Autodesk Inventor part; units mm, degrees
ref_plane "YZ Plane" through (0, 0, 0) normal (1, 0, 0) x (0, 1, 0)
ref_plane "XZ Plane" through (0, 0, 0) normal (0, 1, 0) x (-1, 0, 0)
ref_plane "XY Plane" through (0, 0, 0) normal (0, 0, 1) x (1, 0, 0)
sketch "スケッチ1" plane through (0, 0, 0) normal (0, 0, 1) x (1, 0, 0)
  circle A0 centre (0, 0) radius 1.5
  dimension "d0" = 3
extrude "押し出し1" add sketch "スケッチ1" along normal blind 18
sketch "スケッチ2" plane through (0, 0, 0) normal (0, 0, -1) x (-1, 0, 0)
  circle A0 centre (0, 0) radius 2.75
  dimension "d3" = 5.5
extrude "押し出し2" add sketch "スケッチ2" along normal blind 2
fillet "フィレット1" radius 2 1 edges at (2.75, 0, -2)
thread "ねじ1"
properties part number "ネジ鍋m3,18" material "鋼、高強度、低合金"
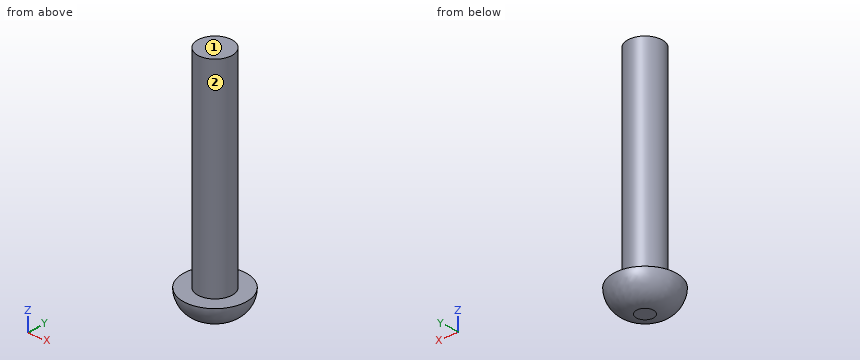
Read the model definition and answer for the solid it produces. Units are mm, in the model's axes. Face numbers are marked on the shaded views. A direction names the side the tool comes from. Coordinates: 2 decimals unless noted, no trailing zeros. Order: outer loops, then holes, each group sorted by start corner. A loop starts at its lowest first (then second) coordinate and runs counter-clockwise, first axis right, second up. Notation, with made-up numbers: (28, 3.25) -> (52, 3.25) arc R33 cw to (52, 38.25) -> close; hole circle Ø1 at (85, -25.5). An arc over 180 degrees is marked (long way). Answer as a JSON object with one key per item and string values.
1) Each of these flat-tipped pins is pushed along its axis until it touches: pin 1 (1 mm diameter, centred on y = 1, z = 7.5, fed in from +X); pin 2 (2 mm diameter, centred on x = -1, z = 5.5, fed in from +Y); pin 3 (1 mm diameter, centred on x = 1, y = -1, fed in from -Z). Where does it stop, or does it pass through?
Model answer:
{"pin 1": "stops at x = 1.41", "pin 2": "stops at y = 1.5", "pin 3": "stops at z = -1.99"}
2) A cutting plane is placed at A-A, the plane z = 2.25. Determine the outline of the cut face in (x, y).
Model answer:
{"outline": "circle Ø3 at (0, 0)"}
3) Consider line 1 along X through (y, z) = (0.05, 12.25); line 2 along Y through (x, z) = (-1.3, 9.75); line 3 along Y through (x, z) = (1.2, 1). Determine where each line is inside the solid, lowest interval first. Write a range as from..to.
Model answer:
{"line 1": "x = -1.5..1.5", "line 2": "y = -0.75..0.75", "line 3": "y = -0.9..0.9"}
4) A tool of negligible diameter and unlimited length cuts with its end or side. For the marked faces 1 and 2, from which of +Z, -Z, +X, -X, +Y, -Y can it reach the whole face along a straight path? Write none if from no direction.
Model answer:
{"face 1": "+Z, +X, -X, +Y, -Y", "face 2": "+Z"}
